Source: CAD feature listing. Evaluate the final solid. Frame: model axes, mm. A direction names the side the tool comes from. Coordinates: 2 decimals unless noted, no trailing zeros. Loops run counter-clockwise (first coordinate to the right, second up) from the corner with the lowest first, then second, coordinate; pieces in that order, holes last. Notation, with made-up numbers: (-13, -13.75) -> (17, -13.75) arc R19 cw to (17, 13.25) -> close; hole circle Ø2 at (32, 79.5). An arc over 180 degrees is marked (long way). Answer as CSV lines item,"result".
from build123d import *

# Parameters (mm, degrees)
ESQUISSE1_R                  = 12
BOSS_EXTRU_1_DEPTH           = 9
ESQUISSE2_R                  = 10
BOSS_EXTRU_2_DEPTH           = 2
ESQUISSE3_R                  = 1.5
ESQUISSE3_R_2                = 2
ENL_V_MAT_EXTRU_1_DEPTH      = 12
ESQUISSE4_R                  = 1.5
ENL_V_MAT_EXTRU_2_DEPTH      = 13
R_P_TITION_CIRCULAIRE1_COUNT = 2
R_P_TITION_CIRCULAIRE1_ANGLE = 90


with BuildPart() as part:
    # Esquisse1 → Boss.-Extru.1 (new body)
    with BuildSketch(Plane.XY):
        Circle(ESQUISSE1_R)
    extrude(amount=BOSS_EXTRU_1_DEPTH)

    # Esquisse2 → Boss.-Extru.2 (add)
    with BuildSketch(Plane.XY.offset(9)):
        Circle(ESQUISSE2_R)
    extrude(amount=BOSS_EXTRU_2_DEPTH)

    # Esquisse3 → Enlèv. mat.-Extru.1 (cut, through all)
    with BuildSketch(Plane.XY.offset(11)):
        with Locations((-5.303300859, -5.303300859)):
            Circle(ESQUISSE3_R)
        with Locations((5.303300859, 5.303300859)):
            Circle(ESQUISSE3_R)
        Circle(ESQUISSE3_R_2)
    extrude(amount=-ENL_V_MAT_EXTRU_1_DEPTH, mode=Mode.SUBTRACT)

    # Esquisse4 → Enlèv. mat.-Extru.2 (cut, through all)
    with BuildSketch(Plane(origin=(0, 0, 0), x_dir=(1, 0, 0), z_dir=(0, 1, 0))):
        with Locations((0, -4.5)):
            Circle(ESQUISSE4_R)
    enl_v_mat_extru_2 = extrude(amount=-ENL_V_MAT_EXTRU_2_DEPTH, mode=Mode.SUBTRACT)

    # Répétition circulaire1: Enlèv. mat.-Extru.2 ×2 about axis
    r_p_tition_circulaire1_axis = Axis((0, 0, 9), (0, 0, 1))
    for i in range(1, R_P_TITION_CIRCULAIRE1_COUNT):
        add(enl_v_mat_extru_2.rotate(r_p_tition_circulaire1_axis, i * R_P_TITION_CIRCULAIRE1_ANGLE / (R_P_TITION_CIRCULAIRE1_COUNT - 1)), mode=Mode.SUBTRACT)


solid = part.part
(1) Pin query (flat end, axial travel): pin 1 Ø5 at (x, z) = (-8.5, 3.5) entering from -Y; pin 2 Ø3 at (x, y) = (0, 0) entering from +Z; pin 3 Ø3 at (y, z) = (-8.5, 7) entering from +X; pin 4 Ø3 at (x, z) = (2.5, 6) entering from -Y. Return the tip coordinate at first contact, or that it passes through.
Computed values:
pin 1,"y = -10.39"
pin 2,"through"
pin 3,"x = 9.75"
pin 4,"y = -11.96"
(2) Cut plane B-B (y = 0). Return the cut outline in (x, z).
Computed values:
outline,"(-12, 0) -> (-2, 0) -> (-2, 11) -> (-10, 11) -> (-10, 9) -> (-12, 9) -> close; (2, 0) -> (12, 0) -> (12, 3) -> (2, 3) -> close; (2, 6) -> (12, 6) -> (12, 9) -> (10, 9) -> (10, 11) -> (2, 11) -> close"
(3) Cut plane C-C (z = 4.5). Return the cut outline in (x, y).
Computed values:
outline,"(-1.5, -11.91) -> (-1.5, -1.32) arc R2 cw to (1.32, 1.5) -> (11.91, 1.5) arc R12 ccw (long way) to start; (1.5, -11.91) arc R12 ccw to (11.91, -1.5) -> (1.5, -1.5) -> close; hole circle Ø3 at (-5.3, -5.3); hole circle Ø3 at (5.3, 5.3)"
(4) Cut plane D-D (y = 6.25). Return the cut outline in (x, z).
Computed values:
outline,"(-10.24, 0) -> (4.14, 0) -> (4.14, 11) -> (-7.81, 11) -> (-7.81, 9) -> (-10.24, 9) -> close; (6.47, 0) -> (10.24, 0) -> (10.24, 9) -> (7.81, 9) -> (7.81, 11) -> (6.47, 11) -> close"
(5) Draft query along Y for faces 1 (the cylindrical face through (-2.17, -9.76, 9.99)), 2 (the flat face through (-2.4, 0.1, 11)), 3 (the cylindrical face through (-6.41, -4.29, 5.58)). Return one class per face: released by +Y, released by -Y, zero draft, split by the parting line, or undercut.
Computed values:
face 1,"split by the parting line"
face 2,"zero draft"
face 3,"undercut"
(6) Cut plane A-A (x = 0). Return the cut outline in (y, z), then the cut area to 3 significant figures.
Computed values:
outline,"(-12, 0) -> (-2, 0) -> (-2, 3) -> (-12, 3) -> close; (-12, 6) -> (-2, 6) -> (-2, 11) -> (-10, 11) -> (-10, 9) -> (-12, 9) -> close; (2, 0) -> (12, 0) -> (12, 9) -> (10, 9) -> (10, 11) -> (2, 11) -> close"
area,"182 mm^2"
(7) Material intervals for L1, parallel to Z at x = -8.5, y = -6; L2, parallel to X at y = -5.25, z = 7.25; L3, parallel to Y at x = 0.5, z = 1.75, sorted ascending. Write a range as [from, to].
Computed values:
L1,"[0, 9]"
L2,"[-10.79, -6.8], [-3.8, 10.79]"
L3,"[-11.99, -1.94], [1.94, 11.99]"
(8) Access query for faces 4 (the cylindrical face through (7, 0, 3)), 5 (the flat face through (2.5, 0.2, 0)), 6 (the cylindrical face through (4.98, 3.84, 5.58)), 7 (the cylindrical face through (0, -7, 3)), 8 (the flat face through (-5, 9, 9)). Directions: +Z, -Z, +X, -X, +Y, -Y. A direction counts if a zero-diameter tool reaches every point of the face in a straight line with its end or side. Return the directions, or none.
Computed values:
face 4,"+X"
face 5,"-Z, +X, -X, +Y, -Y"
face 6,"+Z, -Z"
face 7,"-Y"
face 8,"+Z"
